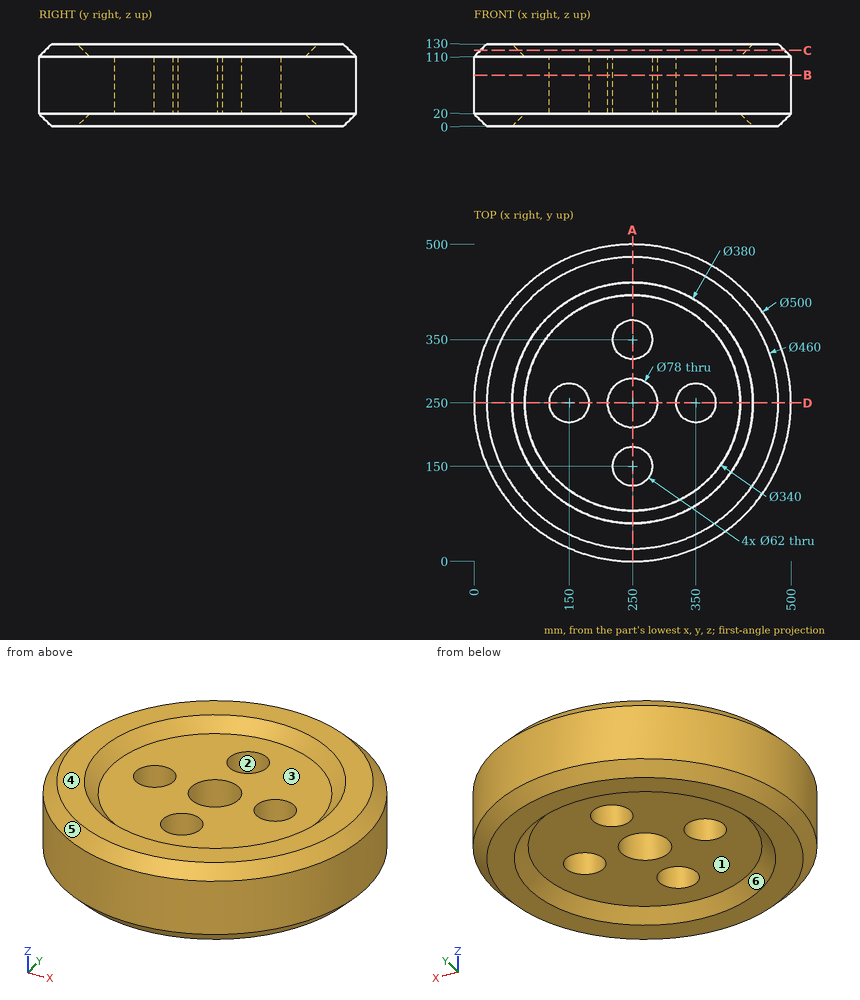
Part print with two shaded views. Sizes in mm from the minimum x, y, z corner. A direction names the side the tool comes from. Coordinates: 2 decimals unless noted, no trailing zeros. Write each loop counter-clockwise with the first axis right and the second up, starting at its lowest first coordinate (ties: lowest second). Pieces come first, ordered by that corner, then holes.
(1) Cut at C-C on z = 120. List the corners of the cut face in (x, y).
(2) 3-axis set-ups, long thin cutter, end or side, ignore diameter. For the marked faces 1, 2 and 3: which of +Z, -Z, +X, -X, +Y, -Y reach the whole face in a straight line?
(3) Cut at A-A on x = 250. List the corners of the cut face in (y, z), and give its area (3 significant figures).
(4) Mould opens along Y. For the marked faces 4, 5 and 6 say: pulls with the +Y half, pulls with the -Y half, needs draft (parallel to the pull), parting line crosses it, or undercut.
(5) Cut at B-B on z = 81. List the corners of the cut face in (x, y).
(6) Pin check, flat tips, straight feed: pin 1 Ø12 at (x, y) = (406, 210) entering from -Z; pin 2 Ø6 at (x, z) = (53.5, 46) entering from +Y; pin 3 Ø8 at (y, z) = (438, 115) entering from +X. Stop position of each tip, or through.
(7) Cut at D-D on y = 250. State how many separate pieces and enclosed holes the cut face has, and give its area (3 significant figures).
(8) Drill centre lines: line 1 (Y direction, x = 250, z = 40.5); line 2 (X direction, y = 143.5, z = 42); line 3 (Y direction, x = 142.5, z = 9.5). Where is each one in solid material? Low to high.
Working result:
1. outline: circle Ø480 at (250, 250); hole circle Ø360 at (250, 250)
2. face 1: -Z
2. face 2: +Z, -Z
2. face 3: +Z
3. outline: (0, 20) - (20, 0) - (60, 0) - (80, 20) - (119, 20) - (119, 110) - (80, 110) - (60, 130) - (20, 130) - (0, 110) - close; (181, 20) - (211, 20) - (211, 110) - (181, 110) - close; (289, 20) - (319, 20) - (319, 110) - (289, 110) - close; (381, 20) - (420, 20) - (440, 0) - (480, 0) - (500, 20) - (500, 110) - (480, 130) - (440, 130) - (420, 110) - (381, 110) - close
3. area: 31,600 mm2
4. face 4: needs draft
4. face 5: parting line crosses it
4. face 6: undercut
5. outline: circle Ø500 at (250, 250); hole circle Ø62 at (150, 250); hole circle Ø78 at (250, 250); hole circle Ø62 at (250, 150); hole circle Ø62 at (250, 350); hole circle Ø62 at (350, 250)
6. pin 1: stops at z = 20
6. pin 2: stops at y = 408.3
6. pin 3: stops at x = 414.79
7. separate pieces: 4
7. enclosed holes: 0
7. area: 31,600 mm2
8. line 1: y = 0 to 119, 181 to 211, 289 to 319, 381 to 500
8. line 2: x = 23.82 to 219.69, 280.31 to 476.18
8. line 3: y = 35.98 to 105, 395 to 464.02
